Geometry: final body of the model. Coordinates: model frame, mm. A direction names the side the tool comes from. Give positions to 0.01 mm unless a question says otherwise; leave off trailing zeros. Write each loop counter-clockwise with the first axis right and the second up, starting at its lowest first coordinate (ties: lowest second). Pieces come first, ordered by that corner, then holes.
from build123d import *

# Parameters (mm, degrees)
SKETCH_1_R          = 2.85
EXTRUDE_1_DEPTH     = 3
SKETCH_2_R          = 1.5
EXTRUDE_2_DEPTH     = 8
FILLET_1_R          = 0.3
CUT_EXTRUDE_1_DEPTH = 1.5


with BuildPart() as part:
    # 草图1 → 凸台-拉伸1 (new body)
    with BuildSketch(Plane(origin=(0, 0, 0), x_dir=(1, 0, 0), z_dir=(0, 1, 0))):
        with Locations(Location((0, 0, 0), (0, 0, 270))):
            Circle(SKETCH_1_R)
    extrude(amount=EXTRUDE_1_DEPTH)

    # 草图2 → 凸台-拉伸2 (add)
    with BuildSketch(Plane.XZ):
        with Locations(Location((0, 0, 0), (0, 0, 90))):
            Circle(SKETCH_2_R)
    extrude(amount=EXTRUDE_2_DEPTH)

    # 圆角1
    fillet_1_edges = [part.edges().sort_by_distance(p)[0] for p in [
        (0, 0, -2.85),
        (0, 3, -2.85),
    ]]
    fillet(fillet_1_edges, radius=FILLET_1_R)

    # 草图3 → 切除-拉伸1 (cut)
    with BuildSketch(Plane(origin=(0, 3, 0), x_dir=(1, 0, 0), z_dir=(0, 1, 0))):
        Polygon((-1.443375673, 0), (-0.721687836, -1.25), (0.721687836, -1.25), (1.443375673, 0), (0.721687836, 1.25), (-0.721687836, 1.25), align=None)
    extrude(amount=-CUT_EXTRUDE_1_DEPTH, mode=Mode.SUBTRACT)


solid = part.part
Q1. Section C-C on y = -7. Output: boundary loops of the cut face in (x, z).
Filled sheet:
outline: circle Ø3 at (0, 0)
Q2. Access query for faces 4 (the flat face through (-1.1, 3, 1.1)), 5 (the flat face through (0, 2, 1.25)), 6 (the flat face through (-2, 0, 0)). Directions: +Z, -Z, +X, -X, +Y, -Y. A direction counts if a zero-diameter tool reaches every point of the face in a straight line with its end or side. Return the directions, or none.
Filled sheet:
face 4: +Z, -Z, +X, -X, +Y
face 5: +Y
face 6: -Y
Q3. Ray query, line 1 along Y through (x, z) = (-0.7, 0.6); line 2 along Y through (x, z) = (1.8, 0.5); line 3 along X through (y, z) = (-2, 0.4). Return the intervals inside material, ascending.
Filled sheet:
line 1: y = -8 to 1.5
line 2: y = 0 to 3
line 3: x = -1.45 to 1.45
Q4. Pull-direction query (X, two-part tool) for faces 1 (the flat face through (0, -8, 0)), 2 (the cylindrical face through (-1.734, 1.483, -2.262)), 3 (the flat face through (0, 2, -1.25)); classes: released by +X, released by -X, zero draft, split by the parting line, or undercut.
Filled sheet:
face 1: zero draft
face 2: split by the parting line
face 3: undercut
Q5. Section D-D on y = 0.75. Output: boundary loops of the cut face in (x, z).
Filled sheet:
outline: circle Ø5.7 at (0, 0)
Q6. Section B-B on x = 0. Output: boundary loops of the cut face in (y, z), plus the area to 3 significant figures.
Filled sheet:
outline: (-8, -1.5) - (0, -1.5) - (0, -2.55) arc R0.3 ccw to (0.3, -2.85) - (2.7, -2.85) arc R0.3 ccw to (3, -2.55) - (3, -1.25) - (1.5, -1.25) - (1.5, 1.25) - (3, 1.25) - (3, 2.55) arc R0.3 ccw to (2.7, 2.85) - (0.3, 2.85) arc R0.3 ccw to (0, 2.55) - (0, 1.5) - (-8, 1.5) - close
area: 37.3 mm2
Q7. Section A-A on y = 2. Output: boundary loops of the cut face in (x, z).
Filled sheet:
outline: circle Ø5.7 at (0, 0); hole (-1.44, 0) - (-0.72, -1.25) - (0.72, -1.25) - (1.44, 0) - (0.72, 1.25) - (-0.72, 1.25) - close
Q8. Pin query (flat end, axial travel): P1, Ø1.5, axis at x = 1.5, y = -3.5, coming from the +Z side; P2, Ø3, axis at y = -4, z = -0.5, coming from the -X side; P3, Ø1.2, axis at x = -0.5, z = 0, coming from the +Y side. Return the tip coordinate at first contact, or that it passes through.
Filled sheet:
P1: stops at z = 1.3
P2: stops at x = -1.5
P3: stops at y = 1.5
